```python
from build123d import *

# Parameters (mm, degrees)
SKETCH002_W          = 34
SKETCH002_H          = 4
PAD001_DEPTH         = 30
EXTRUSION008_DEPTH   = 13.9308213426
BOX003_W             = 13
BOX003_H             = 10
BOX003_DEPTH         = 60
FACE006_W            = 8.14
FACE006_H            = 69.180787832
EXTRUSION006_DEPTH   = 0.4604923972
EXTRUSION005_DEPTH   = 8.14
FACE003_W            = 4
FACE003_H            = 14
EXTRUSION003_DEPTH   = 3.51
FACE004_W            = 3.51
FACE004_H            = 4
EXTRUSION004_DEPTH   = 69.180787832
FACE007_W            = 4
FACE007_H            = 69.180787832
EXTRUSION007_DEPTH   = 0.4131433628
FACE002_W            = 10
FACE002_H            = 4
EXTRUSION002_DEPTH   = 14
EXTRUSION_DEPTH      = 10
EXTRUSION001_DEPTH   = 10
FUSION001_ROLL_ANGLE = 5.0006445976
BOX002_W             = 13
BOX002_H             = 13
BOX002_DEPTH         = 49
BOX001_W             = 15
BOX001_H             = 11
BOX001_DEPTH         = 49
BOX_W                = 31
BOX_H                = 18
BOX_DEPTH            = 14
CYLINDER_R           = 14.5
CYLINDER_DEPTH       = 13
CYLINDER_ROLL_ANGLE  = 90.0000000001
SKETCH_R             = 1
PAD_DEPTH            = 11
CHAMFER_SIZE         = 1
CHAMFER001_SIZE      = 1
CHAMFER002_SIZE      = 1
CHAMFER003_SIZE      = 1
CHAMFER004_SIZE      = 1
CHAMFER005_SIZE      = 1
CHAMFER006_SIZE      = 1
EXTRUSION009_DEPTH   = 13.9308213426
POCKET_DEPTH         = 5
CHAMFER007_SIZE      = 1


with BuildPart() as pad001:
    # Sketch002 → Pad001 (new body)
    with BuildSketch(Plane.YZ):
        with Locations((-15, 58)):
            Rectangle(SKETCH002_W, SKETCH002_H)
    extrude(amount=PAD001_DEPTH)


with BuildPart() as extrusion008:
    # Face008 → Extrusion008 (new body)
    with BuildSketch(Plane(origin=(-17.578899357, -16.0333863028, 53.0614958622), x_dir=(-1, 0, 0), z_dir=(0, -0.9961937175, -0.0871669503))):
        Polygon((4.421100643, -4.5183191267), (4.421100643, -0.5183191267), (1.021100643, -0.5183191267), (1.021100643, 2.4816808733), (1.521100643, 2.9816808733), (1.521100643, 4.9816808733), (0.521100643, 5.9816808733), (-1.978899357, 5.9816808733), (-2.978899357, 4.9816808733), (-2.978899357, -3.5183191267), (-1.978899357, -4.5183191267), align=None)
    extrude(amount=EXTRUSION008_DEPTH)


with BuildPart() as cube003:
    # Box003 → Box003 (new body)
    with BuildSketch(Plane(origin=(-27, 0, 0), x_dir=(1, 0, 0), z_dir=(0, 0, 1))):
        with Locations((6.5, 5)):
            Rectangle(BOX003_W, BOX003_H)
    extrude(amount=BOX003_DEPTH)


with BuildPart() as extrusion006:
    # Face006 → Extrusion006 (new body)
    with BuildSketch(Plane(origin=(-17.93, -18.7549998831, 43.8980956594), x_dir=(-1, 0, 0), z_dir=(0, -0.9961937175, -0.0871669503))):
        Rectangle(FACE006_W, FACE006_H)
    extrude(amount=EXTRUSION006_DEPTH)


with BuildPart() as extrusion005:
    # Face005 → Extrusion005 (new body)
    with BuildSketch(Plane(origin=(-22, -17.0066799089, 44.0510736571), x_dir=(0, -1, 0), z_dir=(1, 0, 0))):
        Polygon((4.7634591209, -34.3057551071), (-1.2668191725, 34.6117111026), (-4.7634591209, 34.3057551071), (1.2668191725, -34.6117111026), align=None)
    extrude(amount=EXTRUSION005_DEPTH)


with BuildPart() as extrusion003:
    # Face003 → Extrusion003 (new body)
    with BuildSketch(Plane(origin=(-24, -15.1296920845, 2.4660065321), x_dir=(-1, 0, 0), z_dir=(0, -0.9961937175, -0.0871669503))):
        Rectangle(FACE003_W, FACE003_H)
    extrude(amount=-EXTRUSION003_DEPTH)


with BuildPart() as fusion002:
    # Face004 → Extrusion004 (new body)
    with BuildSketch(Plane(origin=(-24, -13.9915407622, 9.5923405523), x_dir=(0, 0.9961937175, 0.0871669503), z_dir=(0, -0.0871669503, 0.9961937175))):
        Rectangle(FACE004_W, FACE004_H)
    extrude(amount=EXTRUSION004_DEPTH)

    # Fusion002: union Extrusion003
    add(extrusion003.part)


with BuildPart() as fusion003:
    # Face007 → Extrusion007 (new body)
    with BuildSketch(Plane(origin=(-24, -18.7549998831, 43.8980956594), x_dir=(-1, 0, 0), z_dir=(0, -0.9961937175, -0.0871669503))):
        Rectangle(FACE007_W, FACE007_H)
    extrude(amount=EXTRUSION007_DEPTH)

    # Fusion003: union Extrusion006, Extrusion005, Fusion002
    add(extrusion006.part)
    add(extrusion005.part)
    add(fusion002.part)


with BuildPart() as extrusion002:
    # Face002 → Extrusion002 (new body)
    with BuildSketch(Plane(origin=(-24, -15, 11), x_dir=(0, -1, 0), z_dir=(0, 0, -1))):
        Rectangle(FACE002_W, FACE002_H)
    extrude(amount=EXTRUSION002_DEPTH)


with BuildPart() as extrusion:
    # Face → Extrusion (new body)
    with BuildSketch(Plane(origin=(-22.5493005697, -10, 39.3433444568), x_dir=(-1, 0, 0), z_dir=(0, -1, 0))):
        Polygon((3.4506994303, 28.3433444568), (-0.5493005697, 28.3433444568), (-0.5493005697, -15.6566555432), (-3.9493005697, -15.6566555432), (-3.9493005697, -12.6566555432), (-3.4493005697, -12.1566555432), (-3.4493005697, -10.1566555432), (-4.4493005697, -9.1566555432), (-6.9493005697, -9.1566555432), (-7.9493005697, -10.1566555432), (-7.9493005697, -18.6566555432), (-6.9493005697, -19.6566555432), (2.4506994303, -19.6566555432), (3.4506994303, -18.6566555432), align=None)
    extrude(amount=EXTRUSION_DEPTH)


with BuildPart() as cut005:
    # Face001 → Extrusion001 (new body)
    with BuildSketch(Plane(origin=(-22.5493005697, -10, 39.3433444568), x_dir=(1, 0, 0), z_dir=(0, 1, 0))):
        Polygon((0.5493005697, 28.3433444568), (-3.4506994303, 28.3433444568), (-3.4506994303, -18.6566555432), (-2.4506994303, -19.6566555432), (6.9493005697, -19.6566555432), (7.9493005697, -18.6566555432), (7.9493005697, -10.1566555432), (6.9493005697, -9.1566555432), (4.4493005697, -9.1566555432), (3.4493005697, -10.1566555432), (3.4493005697, -12.1566555432), (3.9493005697, -12.6566555432), (3.9493005697, -15.6566555432), (0.5493005697, -15.6566555432), align=None)
    extrude(amount=EXTRUSION001_DEPTH)

    # Fusion: union Extrusion
    add(extrusion.part)

    # Fusion001: union Extrusion002
    add(extrusion002.part)


with BuildPart() as cut005_1:
    # Fusion001 roll: moved
    add(cut005.part.rotate(Axis((0, 0, 0), (1, 0, 0)), FUSION001_ROLL_ANGLE))


with BuildPart() as cut005_2:
    # Fusion001 placement: moved
    add(cut005_1.part.moved(Location((0, 5.1428500666, 0.2245706677))))

    # Cut004: cut Fusion003
    add(fusion003.part, mode=Mode.SUBTRACT)

    # Cut005: cut Cube003
    add(cube003.part, mode=Mode.SUBTRACT)


with BuildPart() as cube002:
    # Box002 → Box002 (new body)
    with BuildSketch(Plane(origin=(-27, -12, 11), x_dir=(1, 0, 0), z_dir=(0, 0, 1))):
        with Locations((6.5, 6.5)):
            Rectangle(BOX002_W, BOX002_H)
    extrude(amount=BOX002_DEPTH)


with BuildPart() as cube001:
    # Box001 → Box001 (new body)
    with BuildSketch(Plane(origin=(-29, -21, 11), x_dir=(1, 0, 0), z_dir=(0, 0, 1))):
        with Locations((7.5, 5.5)):
            Rectangle(BOX001_W, BOX001_H)
    extrude(amount=BOX001_DEPTH)


with BuildPart() as cube:
    # Box → Box (new body)
    with BuildSketch(Plane(origin=(-15, -23, -3), x_dir=(1, 0, 0), z_dir=(0, 0, 1))):
        with Locations((15.5, 9)):
            Rectangle(BOX_W, BOX_H)
    extrude(amount=BOX_DEPTH)


with BuildPart() as cylinder:
    # Cylinder → Cylinder (new body)
    with BuildSketch(Plane.XY):
        Circle(CYLINDER_R)
    extrude(amount=CYLINDER_DEPTH)


with BuildPart() as cylinder_1:
    # Cylinder roll: moved
    add(cylinder.part.rotate(Axis((0, 0, 0), (1, 0, 0)), CYLINDER_ROLL_ANGLE))


with BuildPart() as cylinder_2:
    # Cylinder placement: moved
    add(cylinder_1.part.moved(Location((0, 1, 12))))


with BuildPart() as fusion004:
    # Sketch → Pad (new body)
    with BuildSketch(Plane.XZ):
        Polygon((15, -7), (15, 3), (-22, 3), (-22, 55), (-18.6, 55), (-18.6, 52), (-19.1, 51.5), (-19.1, 48.5), (-14.6, 48.5), (-14.6, 59), (-26, 59), (-26, -7), align=None)
        with Locations((-12, 0)):
            Circle(SKETCH_R, mode=Mode.SUBTRACT)
        with Locations((12, 0)):
            Circle(SKETCH_R, mode=Mode.SUBTRACT)
    extrude(amount=PAD_DEPTH)

    # Cut: cut Cylinder
    add(cylinder_2.part, mode=Mode.SUBTRACT)

    # Cut001: cut Cube
    add(cube.part, mode=Mode.SUBTRACT)

    # Chamfer
    chamfer_edges = [fusion004.edges().sort_by_distance(p)[0] for p in [
        (15, -5.5, -7),
    ]]
    chamfer(chamfer_edges, length=CHAMFER_SIZE)

    # Chamfer001
    chamfer001_edges = [fusion004.edges().sort_by_distance(p)[0] for p in [
        (-26, -5.5, -7),
    ]]
    chamfer(chamfer001_edges, length=CHAMFER001_SIZE)

    # Chamfer002
    chamfer002_edges = [fusion004.edges().sort_by_distance(p)[0] for p in [
        (-26, -5.5, 59),
    ]]
    chamfer(chamfer002_edges, length=CHAMFER002_SIZE)

    # Chamfer003
    chamfer003_edges = [fusion004.edges().sort_by_distance(p)[0] for p in [
        (-14.6, -5.5, 59),
    ]]
    chamfer(chamfer003_edges, length=CHAMFER003_SIZE)

    # Chamfer004
    chamfer004_edges = [fusion004.edges().sort_by_distance(p)[0] for p in [
        (-14.6, -5.5, 48.5),
    ]]
    chamfer(chamfer004_edges, length=CHAMFER004_SIZE)

    # Chamfer005
    chamfer005_edges = [fusion004.edges().sort_by_distance(p)[0] for p in [
        (-19.1, -5.5, 48.5),
    ]]
    chamfer(chamfer005_edges, length=CHAMFER005_SIZE)

    # Chamfer006
    chamfer006_edges = [fusion004.edges().sort_by_distance(p)[0] for p in [
        (15, -2.5, 3),
    ]]
    chamfer(chamfer006_edges, length=CHAMFER006_SIZE)

    # Cut002: cut Cube001
    add(cube001.part, mode=Mode.SUBTRACT)

    # Cut003: cut Cube002
    add(cube002.part, mode=Mode.SUBTRACT)

    # Fusion004: union Cut005
    add(cut005_2.part)


with BuildPart() as chamfer007:
    # Face009 → Extrusion009 (new body)
    with BuildSketch(Plane(origin=(-23.9956483899, -14.3298412993, 33.5924101077), x_dir=(-1, 0, 0), z_dir=(0, -0.9961937175, -0.0871669503))):
        Polygon((2.0043516101, 23.9382071366), (-1.9956483899, 23.9382071366), (-1.9956483899, -20.0617928634), (-1.9956483899, -24.0617928634), (1.0043516101, -24.0617928634), (2.0043516101, -23.0617928634), align=None)
    extrude(amount=EXTRUSION009_DEPTH)

    # Sketch001 → Pocket (cut)
    with BuildSketch(Plane.YZ.offset(-22)):
        Polygon((-12.153362, 9.710751), (-30, 47.063831), (-30, 0), align=None)
    extrude(amount=-POCKET_DEPTH, mode=Mode.SUBTRACT)

    # Fusion005: union Extrusion008, Fusion004
    add(extrusion008.part)
    add(fusion004.part)


with BuildPart() as chamfer007_1:
    # Fusion005 placement: moved
    add(chamfer007.part.moved(Location((30, 0, 0))))

    # Cut006: cut Pad001
    add(pad001.part, mode=Mode.SUBTRACT)

    # Chamfer007
    chamfer007_edges = [chamfer007_1.edges().sort_by_distance(p)[0] for p in [
        (4, -11.406738, 56),
        (15.4, -11.406738, 56),
    ]]
    chamfer(chamfer007_edges, length=CHAMFER007_SIZE)


solid = chamfer007_1.part
```
Design review of the part built by this model. Coordinates are the model's own, in mm. A direction names the side the tool comes from. Coordinates: 2 decimals unless noted, no trailing zeros. Order: outer loops, then holes, each group sorted by start corner. A loop starts at its lowest first (then second) coordinate and runs counter-clockwise, first axis right, second up.
1) Clearance check with flat-ended pins moving along their axes: pin 1 (11 mm diameter, centred on x = 20.5, z = -2.5, fed in from -Y); pin 2 (4 mm diameter, centred on y = -14.5, z = 4, fed in from -X); pin 3 (5 mm diameter, centred on x = 32.5, y = -9.5, fed in from +Z); pin 4 (15 mm diameter, centred on y = -14.5, z = 33.5, fed in from +X). State where each tip first meets the part, or that it passes through.
2) Take a section at A-A, the plane y = -2.5. Give the boundary of the cut face in (x, z), and give its area (3 significant figures).
3) Mouldability with a two-part tool opening along X and no side actions: class faces 1 (the cylindrical face through (43, -2, 0)), 2 (the cylindrical face through (29.8, -2.5, -2.5)), 3 (the flat face through (7.7, 0, 13)), 4 (the flat face through (45, -4, -3)) as +X half, -X half, draft (parallel to the pull), parting line (faces both ways), or undercut.
4) For faces 5 (the flat face through (12, -5, 3)), 6 (the flat face through (15, -8, 0)), 7 (the flat face through (10.9, -15, 49)), list the 3-axis set-ups (+Z, -Z, +X, -X, +Y, -Y) from which the entire face can be reached by the end or side of a thin tool; tool diameter is ignored.
5) Take a section at C-C, the plane x = 21. Give the boundary of the cut face in (y, z).
6) Take a section at B-B, the plane z = 0. Give the boundary of the cut face in (x, y).
7) Take a section at D-D, the plane y = -24. Give the boundary of the cut face in (x, z), and give its area (3 significant figures).
8) Wall thickness on line 1 along X through (y, z) = (-8.5, 50); line 2 along Z through (x, y) = (18, -1.1); line 3 along X through (y, z) = (-16, 44.5): over which ranges is each line inside the solid? List them lowest first.
Returned:
1. pin 1: stops at y = -11
1. pin 2: passes through
1. pin 3: stops at z = -3
1. pin 4: stops at x = 8
2. outline: (4, -6) - (5, -7) - (44, -7) - (45, -6) - (45, 2) - (44, 3) - (41.37, 3) arc R14.5 cw to (18.63, 3) - (8, 3) - (8, 54.77) - (11.4, 54.77) - (11.4, 51.75) - (10.9, 51.25) - (10.9, 49.24) - (11.9, 48.24) - (14.4, 48.24) - (15.4, 49.24) - (15.4, 55) - (14.4, 56) - (5, 56) - (4, 55) - close; hole circle Ø2 at (18, 0); hole circle Ø2 at (42, 0)
2. area: 562 mm2
3. face 1: undercut
3. face 2: undercut
3. face 3: draft
3. face 4: +X half
4. face 5: +X, +Y, -Y
4. face 6: +X, -Y
4. face 7: +Y, -Y
5. outline: (-11, -7) - (0, -7) - (0, 0.63) - (-5, 0.63) - (-5, -3) - (-11, -3) - close
6. outline: (4, -11.39) - (8, -11.39) - (8, -11) - (15, -11) - (15, -5) - (17, -5) - (17, 0) - (4, 0) - close; (19, -5) - (21.86, -5) - (21.86, 0) - (19, 0) - close; (38.14, -5) - (41, -5) - (41, 0) - (38.14, 0) - close; (43, -5) - (45, -5) - (45, 0) - (43, 0) - close
7. outline: (4, 34.51) - (8, 34.51) - (8, 52.88) - (11.4, 52.88) - (11.4, 49.87) - (10.9, 49.37) - (10.9, 47.36) - (11.9, 46.36) - (14.4, 46.36) - (15.4, 47.36) - (15.4, 55) - (14.4, 56) - (5, 56) - (4, 55) - close
7. area: 135 mm2
8. line 1: x = 4 to 8, 10.9 to 15.4
8. line 2: z = -7 to -1, 1 to 3
8. line 3: x = 4 to 8
